Input: part model. Units: mm. Frame: model coordinates. Face numbers are marked on the shaded views. Round coordinates to 2 decimals unless told otherwise and drop trailing zeros. Loops run counter-clockwise (first coordinate to the right, second up) from the corner with the lowest first, then second, coordinate; pieces in that order, holes last. Notation, with made-up numbers: M 54.5,32 L 113.5,32 A24 ccw 113.5,54 Z; hole C 60,14 d4. An arc over 180 degrees is marked long. Put each result on its own line as item: value. Start each with the question number.
1) Pin query (flat end, axial travel): pin 1 (0.6 mm diameter, centred on x = 66, z = -5, fed in from +Y); pin 2 (0.6 mm diameter, centred on x = 66, z = 2, fed in from -Y); pin 3 (2 mm diameter, centred on x = 9, y = 64.5, fed in from +Z); pin 4 (15.5 mm diameter, centred on x = -24, z = 3, fed in from -Y). Return the tip coordinate at first contact, or that it passes through.
2) Draft query along Z for the marked faces 1, 2 and 3. Return one class per face: +Z half, -Z half, draft (parallel to the pull), parting line (faces both ways), or undercut.
3) Section D-D on x = 4.5. Output: boundary loops of the cut face in (y, z), plus the area to 3 significant figures.
4) Section A-A on x = 51.5. Output: boundary loops of the cut face in (y, z).
5) Line query: probe 1 along Z at (x, y) = (33, 46.5); probe 2 along Y at (x, z) = (-11, -16); probe 3 along X at (y, z) = (29, -14). Output: solid intervals per line, ascending.
6) Section C-C on z = 4. State how many separate pieces and enclosed holes the cut face has, plus the area to 3 significant figures.
7) Section B-B on y = 42. Output: boundary loops of the cut face in (x, z).
from build123d import *

# Parameters (mm, degrees)
F0_W         = 130
F0_H         = 130
F1_DEPTH     = 17.5
F2_W         = 126
F2_H         = 31
F3_DEPTH     = 126
F5_DEPTH     = 5
F7_DEPTH     = 3
F9_W         = 122.3782406645
F9_H         = 23.2565429012
F10_DEPTH    = 7
F8_W         = 119.2743226562
F8_H         = 26.0036256061
F11_DEPTH    = 130
F12_T1_DEPTH = 50


# Not quite as in the source:
# - a fillet or chamfer that OpenCascade refuses, or shapes differently, is made with other operations: its cross-section is extruded or revolved along the edge and cut away or added


with BuildPart() as f1:
    # F0 (on Top) → F1 (new body, symmetric)
    with BuildSketch(Plane.XY):
        with Locations((2.0031377077, 1.1643140912)):
            Rectangle(F0_W, F0_H)
    extrude(amount=F1_DEPTH, both=True)

    # F2 (on face) → F3 (cut)
    with BuildSketch(Plane.XZ.offset(63.8356859088)):
        with Locations((2.0031377077, 0)):
            Rectangle(F2_W, F2_H)
    extrude(amount=-F3_DEPTH, mode=Mode.SUBTRACT)

    # F4 (on face) → F5 (join)
    with BuildSketch(Plane.XY.offset(17.5)):
        with BuildLine():
            Line((-24.9968622923, -53.8356859088), (-19.9968622923, -53.8356859088))
            ThreePointArc((-19.9968622923, -53.8356859088), (-22.4968622923, -51.3356859088), (-24.9968622923, -53.8356859088))
        make_face()
        with BuildLine():
            ThreePointArc((-24.9968622923, -53.8356859088), (-22.4968622923, -56.3356859088), (-19.9968622923, -53.8356859088))
            Line((-19.9968622923, -53.8356859088), (-24.9968622923, -53.8356859088))
        make_face()
        with BuildLine():
            ThreePointArc((-19.9968622923, 56.1643140912), (-22.4968622923, 58.6643140912), (-24.9968622923, 56.1643140912))
            Line((-24.9968622923, 56.1643140912), (-19.9968622923, 56.1643140912))
        make_face()
        with BuildLine():
            Line((-19.9968622923, 56.1643140912), (-24.9968622923, 56.1643140912))
            ThreePointArc((-24.9968622923, 56.1643140912), (-22.4968622923, 53.6643140912), (-19.9968622923, 56.1643140912))
        make_face()
        with BuildLine():
            Line((20.0031377077, 56.1643140912), (25.0031377077, 56.1643140912))
            ThreePointArc((25.0031377077, 56.1643140912), (22.5031377077, 58.6643140912), (20.0031377077, 56.1643140912))
        make_face()
        with BuildLine():
            ThreePointArc((20.0031377077, 56.1643140912), (22.5031377077, 53.6643140912), (25.0031377077, 56.1643140912))
            Line((25.0031377077, 56.1643140912), (20.0031377077, 56.1643140912))
        make_face()
        with BuildLine():
            Line((25.0031377077, -53.8356859088), (20.0031377077, -53.8356859088))
            ThreePointArc((20.0031377077, -53.8356859088), (22.5031377077, -56.3356859088), (25.0031377077, -53.8356859088))
        make_face()
        with BuildLine():
            ThreePointArc((25.0031377077, -53.8356859088), (22.5031377077, -51.3356859088), (20.0031377077, -53.8356859088))
            Line((20.0031377077, -53.8356859088), (25.0031377077, -53.8356859088))
        make_face()
        with BuildLine():
            ThreePointArc((54.5031400741, 56.1643140912), (55.2365873133, 54.3987711796), (57.0031377077, 53.6677538545))
            Line((57.0031377077, 53.6677538545), (57.0031377077, 56.1643140912))
            Line((57.0031377077, 56.1643140912), (54.5031400741, 56.1643140912))
        make_face()
        with BuildLine():
            Line((57.0031377077, 56.1643140912), (57.0031377077, 53.6677538545))
            ThreePointArc((57.0031377077, 53.6677538545), (58.7709046607, 54.3999869016), (59.5031377077, 56.1677538545))
            ThreePointArc((59.5031377077, 56.1677538545), (57.0014178256, 58.6677532629), (54.5031400741, 56.1643140912))
            Line((54.5031400741, 56.1643140912), (57.0031377077, 56.1643140912))
        make_face()
        with BuildLine():
            ThreePointArc((57.0031377077, -51.3110916167), (55.2314275833, -52.0546307181), (54.51056035, -53.8356859088))
            Line((54.51056035, -53.8356859088), (57.0031377077, -53.8356859088))
            Line((57.0031377077, -53.8356859088), (57.0031377077, -51.3110916167))
        make_face()
        with BuildLine():
            Line((57.0031377077, -53.8356859088), (54.51056035, -53.8356859088))
            ThreePointArc((54.51056035, -53.8356859088), (57.0227418926, -56.311050683), (59.5104392663, -53.8110809541))
            ThreePointArc((59.5104392663, -53.8110809541), (58.7756228408, -52.0407343925), (57.0031377077, -51.3110916167))
            Line((57.0031377077, -51.3110916167), (57.0031377077, -53.8356859088))
        make_face()
        with BuildLine():
            ThreePointArc((-50.4950310388, -53.8363249032), (-50.4950310593, -53.836005406), (-50.4950311205, -53.8356859088))
            Line((-50.4950311205, -53.8356859088), (-52.9968622923, -53.8356859088))
            Line((-52.9968622923, -53.8356859088), (-52.9968622923, -51.3363255739))
            ThreePointArc((-52.9968622923, -51.3363255739), (-54.7621504273, -55.6047391835), (-50.4950310388, -53.8363249032))
        make_face()
        with BuildLine():
            Line((-52.9968622923, -53.8356859088), (-50.4950311205, -53.8356859088))
            ThreePointArc((-50.4950311205, -53.8356859088), (-51.2281376662, -52.0676848015), (-52.9968622923, -51.3363255739))
            Line((-52.9968622923, -51.3363255739), (-52.9968622923, -53.8356859088))
        make_face()
        with BuildLine():
            Line((-52.9968622923, 56.1643140912), (-52.9968622923, 53.6671405204))
            ThreePointArc((-52.9968622923, 53.6671405204), (-51.2364160366, 54.4018236777), (-50.506650387, 56.1643140912))
            Line((-50.506650387, 56.1643140912), (-52.9968622923, 56.1643140912))
        make_face()
        with BuildLine():
            ThreePointArc((-50.5066488108, 56.1671213651), (-54.777872441, 57.9314248684), (-52.9968622923, 53.6671405204))
            Line((-52.9968622923, 53.6671405204), (-52.9968622923, 56.1643140912))
            Line((-52.9968622923, 56.1643140912), (-50.506650387, 56.1643140912))
            ThreePointArc((-50.506650387, 56.1643140912), (-50.5066492049, 56.1657177279), (-50.5066488108, 56.1671213651))
        make_face()
    extrude(amount=F5_DEPTH)

    # F6 (on face) → F7 (cut)
    with BuildSketch(Plane(origin=(0, 0, -17.5), x_dir=(1, 0, 0), z_dir=(0, 0, -1))):
        Polygon((57.0031377077, 0.8356859088), (2.0031377077, 53.8356859088), (-13.8737854376, 38.5361054233), (22.9762229292, 0.2955307031), (-16.0963200722, -37.3561925527), (2.0758649804, -56.1643140912), align=None)
        Polygon((-35.0628468777, 18.1175553083), (-52.9968622923, 0.8356859088), (-36.3205869987, -16.424176437), (-18.4094090927, 0.8356859088), align=None)
    extrude(amount=-F7_DEPTH, mode=Mode.SUBTRACT)

    # F9 (on face) → F10 (cut)
    with BuildSketch(Plane(origin=(0, 66.1643140912, 0), x_dir=(-1, 0, 0), z_dir=(0, 1, 0))):
        with Locations((-2.0031377077, 0)):
            Rectangle(F9_W, F9_H)
    extrude(amount=-F10_DEPTH, mode=Mode.SUBTRACT)

    # F8 (on face) → F11 (cut)
    with BuildSketch(Plane(origin=(-62.9968622923, 0, 0), x_dir=(0, -1, 0), z_dir=(-1, 0, 0))):
        with Locations((-1.2152138836, -0.0606838628)):
            Rectangle(F8_W, F8_H)
    extrude(amount=-F11_DEPTH, mode=Mode.SUBTRACT)

    # F12: fillet of radius 3 on 4 edges, made by hand

    # F12_s2 → F12_t1 (cut)
    with BuildSketch(Plane.XY.offset(-25)):
        with BuildLine():
            add(Edge.make_bspline(
                [(-59.9968622923, 66.1643140912), (-62.9968622923, 66.1643140912), (-62.9968622923, 63.1643140912)],
                knots=[0, 0, 0, 1, 1, 1], degree=2, weights=[1, 1, 1]))
            Line((-62.9968622923, 63.1643140912), (-62.9968622923, 66.1643140912))
            Line((-62.9968622923, 66.1643140912), (-59.9968622923, 66.1643140912))
        make_face()
        with BuildLine():
            add(Edge.make_bspline(
                [(-62.9968622923, -60.8356859088), (-62.9968622923, -63.8356859088), (-59.9968622923, -63.8356859088)],
                knots=[0, 0, 0, 1, 1, 1], degree=2, weights=[1, 1, 1]))
            Line((-59.9968622923, -63.8356859088), (-62.9968622923, -63.8356859088))
            Line((-62.9968622923, -63.8356859088), (-62.9968622923, -60.8356859088))
        make_face()
        with BuildLine():
            add(Edge.make_bspline(
                [(64.0031377077, 66.1643140912), (67.0031377077, 66.1643140912), (67.0031377077, 63.1643140912)],
                knots=[0, 0, 0, 1, 1, 1], degree=2, weights=[1, 1, 1]))
            Line((67.0031377077, 63.1643140912), (67.0031377077, 66.1643140912))
            Line((67.0031377077, 66.1643140912), (64.0031377077, 66.1643140912))
        make_face()
        with BuildLine():
            add(Edge.make_bspline(
                [(67.0031377077, -60.8356859088), (67.0031377077, -63.8356859088), (64.0031377077, -63.8356859088)],
                knots=[0, 0, 0, 1, 1, 1], degree=2, weights=[1, 1, 1]))
            Line((64.0031377077, -63.8356859088), (67.0031377077, -63.8356859088))
            Line((67.0031377077, -63.8356859088), (67.0031377077, -60.8356859088))
        make_face()
    extrude(amount=F12_T1_DEPTH, mode=Mode.SUBTRACT)


solid = f1.part
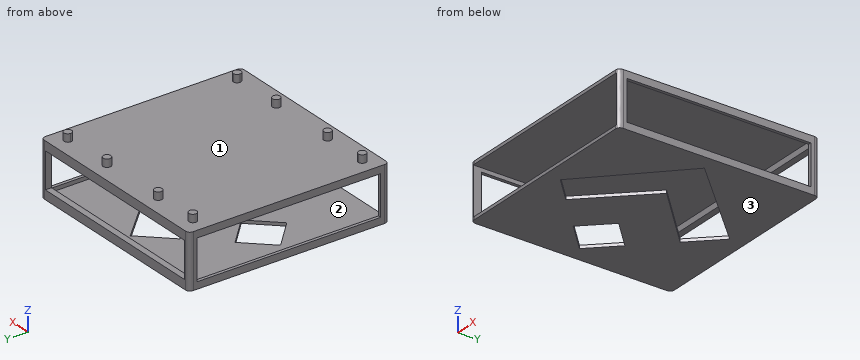
Geometry results:
1. pin 1: stops at y = 65.82
1. pin 2: stops at y = -63.49
1. pin 3: stops at z = 17.5
1. pin 4: passes through
2. face 1: +Z half
2. face 2: undercut
2. face 3: -Z half
3. outline: M -63.84,-17.5 L -51.43,-17.5 L -51.43,-15.5 L -63.84,-15.5 Z; M -63.84,15.5 L 62.16,15.5 L 62.16,11.63 L 66.16,11.63 L 66.16,17.5 L -63.84,17.5 Z; M -19.47,-17.5 L 17.51,-17.5 L 17.51,-15.5 L -19.47,-15.5 Z; M 53.65,-17.5 L 66.16,-17.5 L 66.16,-11.63 L 62.16,-11.63 L 62.16,-15.5 L 53.65,-15.5 Z
3. area: 415 mm²
4. outline: M -63.84,-17.5 L -6.14,-17.5 L -6.14,-15.5 L -63.84,-15.5 Z; M -63.84,15.5 L 62.16,15.5 L 62.16,11.63 L 66.16,11.63 L 66.16,17.5 L -63.84,17.5 Z; M 4.88,-17.5 L 66.16,-17.5 L 66.16,-11.63 L 62.16,-11.63 L 62.16,-15.5 L 4.88,-15.5 Z
5. probe 1: z = -17.5 to -15.5, 15.5 to 17.5
5. probe 2: y = -63.84 to -41.31, -35.55 to 32.45, 42.63 to 66.16
5. probe 3: x = -63 to -61, 65 to 67
6. separate pieces: 4
6. enclosed holes: 0
6. area: 51.5 mm²
7. outline: M -63,-17.5 L -11.61,-17.5 L -11.61,-15.5 L -61,-15.5 L -61,-13.06 L -63,-13.06 Z; M -63,12.94 L -61,12.94 L -61,15.5 L 65,15.5 L 65,12.94 L 67,12.94 L 67,17.5 L -63,17.5 Z; M 15.73,-17.5 L 67,-17.5 L 67,-13.06 L 65,-13.06 L 65,-15.5 L 15.73,-15.5 Z
